```python
from build123d import *

# Parameters (mm, degrees)
F2_R     = 169.8017669699
F2_R_2   = 96.266
F3_DEPTH = 0.5842
F4_R     = 139.446
F4_R_2   = 96.266
F5_DEPTH = 1.0668
F6_SIZE  = 1.524
F7_R     = 35.7886
F7_R_2   = 7.2771
F8_DEPTH = 25.4
F9_SIZE  = 1.524
F10_SIZE = 3.175


with BuildPart() as f1:
    # F0 (on Right) → F1 (revolve)
    with BuildSketch(Plane.YZ):
        Polygon((-5.9944, 0), (0, 0), (0, 82.931), (-19.6342, 82.931), (-19.6342, 139.446), (-31.3944, 139.446), (-31.3944, 77.978), (-5.9944, 77.978), align=None)
    revolve(axis=Axis((0, 54.5056797507, 0), (0, 1, 0)))

    # F2 (on face) → F3 (cut)
    with BuildSketch(Plane(origin=(0, -19.6342, 0), x_dir=(-1, 0, 0), z_dir=(0, 1, 0))):
        Circle(F2_R)
        Circle(F2_R_2, mode=Mode.SUBTRACT)
    extrude(amount=-F3_DEPTH, mode=Mode.SUBTRACT)

    # F4 (on face) → F5 (cut)
    with BuildSketch(Plane.XZ.offset(31.3944)):
        Circle(F4_R)
        Circle(F4_R_2, mode=Mode.SUBTRACT)
    extrude(amount=-F5_DEPTH, mode=Mode.SUBTRACT)

    # F6
    f6_edges = [f1.edges().sort_by_distance(p)[0] for p in [
        (0, -20.2184, -139.446),
        (0, -30.3276, -139.446),
        (0, 0, -82.931),
        (0, -31.3944, -77.978),
    ]]
    chamfer(f6_edges, length=F6_SIZE)

    # F7 (on face) → F8 (cut)
    with BuildSketch(Plane(origin=(0, 0, 0), x_dir=(-1, 0, 0), z_dir=(0, 1, 0))):
        Circle(F7_R)
        with Locations((0, 57.15)):
            Circle(F7_R_2)
        with Locations((-54.3528799063, 17.6603212285)):
            Circle(F7_R_2)
        with Locations((-33.5919271685, -46.2353212285)):
            Circle(F7_R_2)
        with Locations((33.5919271685, -46.2353212285)):
            Circle(F7_R_2)
        with Locations((54.3528799063, 17.6603212285)):
            Circle(F7_R_2)
    extrude(amount=-F8_DEPTH, mode=Mode.SUBTRACT)

    # F9
    f9_edges = [f1.edges().sort_by_distance(p)[0] for p in [
        (7.2771, 0, 57.15),
        (-47.07578, 0, 17.660321),
        (-26.314827, 0, -46.235321),
        (40.869027, 0, -46.235321),
        (61.62998, 0, 17.660321),
        (-26.314827, -5.9944, -46.235321),
        (-47.07578, -5.9944, 17.660321),
        (7.2771, -5.9944, 57.15),
        (61.62998, -5.9944, 17.660321),
        (40.869027, -5.9944, -46.235321),
        (35.7886, 0, 0),
    ]]
    chamfer(f9_edges, length=F9_SIZE)

    # F10
    f10_edges = [f1.edges().sort_by_distance(p)[0] for p in [
        (35.7886, -5.9944, 0),
    ]]
    chamfer(f10_edges, length=F10_SIZE)


solid = f1.part
```
Input: part model. Units: mm. Frame: model coordinates. A direction names the side the tool comes from. Round coordinates to 2 decimals unless told otherwise and drop trailing zeros. Write each loop counter-clockwise with the first axis right and the second up, starting at its lowest first coordinate (ties: lowest second). Pieces come first, ordered by that corner, then holes. Notation, with made-up numbers: (45.5, -29) - (82.5, -29) arc R15 cw to (82.5, -12) - close; hole circle Ø4 at (51, 20). An arc over 180 degrees is marked (long way). Write item = value, one per line.
(1) Pull-direction query (Z, two-part tool) for faces 1 (the conical face through (7.4, -4.6, 57.5)), 2 (the flat face through (-29, -20.218, 94)); classes: +Z half, -Z half, draft (parallel to the pull), parting line (faces both ways), or undercut.
Geometry check:
face_1 = undercut
face_2 = draft
(2) Section query A-A on y = -14. Output: boundary loops of the cut face in (x, z).
Geometry check:
outline = circle Ø165.86 at (0, 0); hole circle Ø155.96 at (0, 0)
(3) Access query for faces 3 (the cylindrical face through (47.412, -2.977, 19.846)), 4 (the flat face through (36, -5.994, 16)). Directions: +Z, -Z, +X, -X, +Y, -Y. A direction counts if a zero-diameter tool reaches every point of the face in a straight line with its end or side. Return the directions, or none.
Geometry check:
face_3 = +Y, -Y
face_4 = -Y
(4) Material intervals for probe 1 along X at (y, z) = (-13.5, 0); probe 2 along Z at (x, y) = (-2, -14); probe 3 along Y at (x, z) = (5, 124.5), sorted ascending.
Geometry check:
probe_1 = -82.93 to -77.98, 77.98 to 82.93
probe_2 = -82.91 to -77.95, 77.95 to 82.91
probe_3 = -30.33 to -20.22
(5) Section query B-B on x = 0. State how many separate pieces and enclosed holes the cut face has, then the cut area to 3 significant figures.
Geometry check:
separate_pieces = 3
enclosed_holes = 0
area = 1,890 mm^2
(6) Contact query for flat-ended pins moving along their axis: pin 1 Ø2 at (x, z) = (30.5, 71.5) entering from +Y; pin 2 Ø2 at (y, z) = (-8.5, -31) entering from -X; pin 3 Ø11.5 at (x, z) = (-33.59, -46.24) entering from +Y; pin 4 Ø1.5 at (x, y) = (25, -13.5) entering from -Z. Output: stop coordinate, or through.
Geometry check:
pin_1 = 0
pin_2 = -77.31
pin_3 = through
pin_4 = -79.31
